Verification items for the finished model (mm, model axes). Face numbers are marked on the shaded views. A direction names the side the tool comes from. Give positions to 0.01 mm unless a question says otherwise; leave off trailing zeros. Order: outer loops, then holes, each group sorted by start corner. A loop starts at its lowest first (then second) coordinate and runs counter-clockwise, first axis right, second up. Notation, with made-up numbers: (-22, 33) - (1, 33) arc R24 ccw to (1, 44) - close; hole circle Ø1 at (-24, 45). An arc over 180 degrees is marked (long way). Answer as a JSON object with one key per item and string values. Group by question number.
(1) Access from +Z, -Z, +X, -X, +Y, -Y to the whole of each face (thin tool, end or side, straight path). Record for the marked faces 1, 2 and 3.
(2) Section check A-A (x = 0). Count the separate pieces of the cut face and the enclosed holes in it, then the cut area to 3 significant figures.
(3) Section check D-D (y = -11.5). Record the boundary of the cut face in (x, z) (3 decimals), then the cut area to 3 significant figures.
(4) Section check B-B (z = -20). Record the boundary of the cut face in (x, y), then the cut area to 3 significant figures.
(5) Thickness scan on line 1 (Y direction, x = 11.5, z = -27); line 2 (X direction, y = -20, z = 8); line 3 (Y direction, x = 0, z = 22.25). Record the ranges inside material, lowest first.
(6) Mould release check, pull along Z, two halves, no side actions. Record for the marked faces 4, 5 and 6: +Z half, -Z half, draft (parallel to the pull), parting line (faces both ways), or undercut.
(7) Depth check by flat-ended pin: pin 1 Ø5 at (x, y) = (1.5, 26.5) entering from -Z; pin 2 Ø2 at (x, z) = (-19, -17) entering from +Y; pin 3 Ø4 at (y, z) = (-24.5, 23) entering from -X; pin 4 Ø16 at (x, z) = (0, 8) entering from +Y. Enter the tip coordinate at first touch or a pass-through.
```python
from build123d import *

# Parameters (mm, degrees)
F0_W          = 44
F0_H          = 60
F1_DEPTH      = 24
F2_R          = 21.99999
F3_W          = 34
F3_H          = 54
F4_DEPTH      = 10
F4_DEPTH_BACK = 54
F5_R          = 14
F5_W          = 32
F5_H          = 14
F6_DEPTH      = 48.001
F8_R          = 10
F8_W          = 20
F8_H          = 6
F9_DEPTH      = 64.001
F7_R          = 4
F10_DEPTH     = 7.8348487101


# Not quite as in the source:
# - a fillet or chamfer is up to 0.001 mm smaller than in the source, because OpenCascade refuses the exact size


with BuildPart() as f1:
    # F0 (on Right) → F1 (new body, symmetric)
    with BuildSketch(Plane.YZ):
        Rectangle(F0_W, F0_H)
    extrude(amount=F1_DEPTH, both=True)

    # F2 (radius 22 in the source; OpenCascade refuses exactly that, so slightly less here)
    f2_edges = [f1.edges().sort_by_distance(p)[0] for p in [
        (0, -22, 30),
        (0, 22, 30),
    ]]
    fillet(f2_edges, radius=F2_R)

    # F3 (on face) → F4 (join, two sides)
    with BuildSketch(Plane.XZ.offset(22)) as f4_sk:
        with Locations((0, -3)):
            Rectangle(F3_W, F3_H)
    extrude(amount=F4_DEPTH)
    extrude(f4_sk.sketch, amount=-F4_DEPTH_BACK)

    # F5 (on face) → F6 (cut, through all)
    with BuildSketch(Plane.YZ.offset(24)):
        with Locations((0, 8)):
            Circle(F5_R)
        with Locations((0, -23)):
            Rectangle(F5_W, F5_H)
    extrude(amount=-F6_DEPTH, mode=Mode.SUBTRACT)

    # F8 (on face) → F9 (cut, through all)
    with BuildSketch(Plane.XZ.offset(32)):
        with Locations((0, 8)):
            Circle(F8_R)
        with Locations((0, -27)):
            Rectangle(F8_W, F8_H)
    extrude(amount=-F9_DEPTH, mode=Mode.SUBTRACT)

    # F7 (on face) → F10 (cut, up to face)
    with BuildSketch(Plane.XY.offset(24)):
        with Locations((0, -25)):
            Circle(F7_R)
        with Locations((0, 25)):
            Circle(F7_R)
    extrude(amount=-F10_DEPTH, mode=Mode.SUBTRACT)


solid = f1.part
```
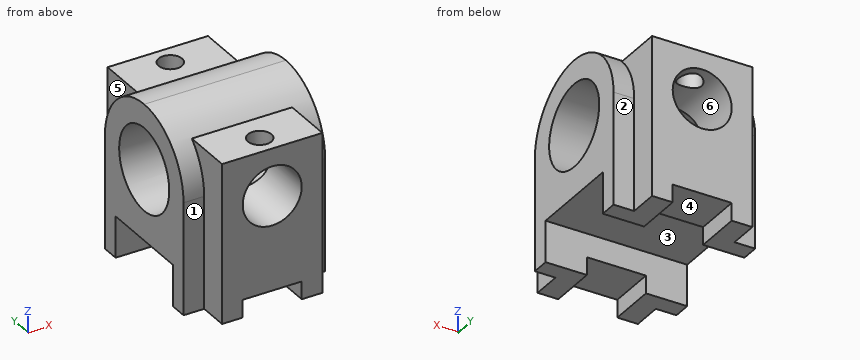
Solutions:
{
 "1": {"face 1": "+Z, -Z, -X, -Y", "face 2": "+Z, -Z, +X, +Y", "face 3": "-Z, +X, -X"},
 "2": {"separate pieces": "4", "enclosed holes": "0", "area": "1,460 mm2"},
 "3": {"outline": "(-24, -16) - (24, -16) - (24, 0.016) - (6.021, 0.016) arc R10 cw to (-6.021, 0.016) - (-24, 0.016) - close; (-24, 15.984) - (-6.021, 15.984) arc R10 cw to (6.021, 15.984) - (24, 15.984) - (24, 26.755) - (-24, 26.755) - close", "area": "1,250 mm2"},
 "4": {"outline": "(-24, -22) - (-17, -22) - (-17, -32) - (17, -32) - (17, -22) - (24, -22) - (24, -16) - (-24, -16) - close; (-24, 16) - (24, 16) - (24, 22) - (17, 22) - (17, 32) - (-17, 32) - (-17, 22) - (-24, 22) - close", "area": "1,260 mm2"},
 "5": {"line 1": "y = -32 to -16, 16 to 32", "line 2": "x = -24 to -10, 10 to 24", "line 3": "y = -32 to -29, -21 to 21, 29 to 32"},
 "6": {"face 4": "-Z half", "face 5": "draft", "face 6": "undercut"},
 "7": {"pin 1": "stops at z = -24", "pin 2": "stops at y = 22", "pin 3": "stops at x = -17", "pin 4": "passes through"}
}
